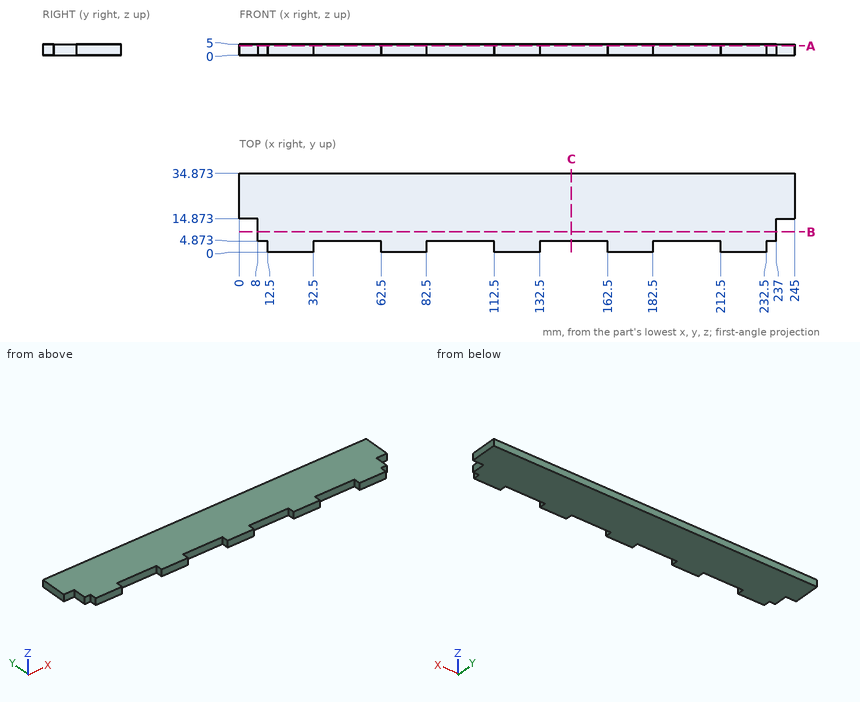
Source: three-view drawing plus pictorial views. Frame: mm from the lowest corner of the part. Give positions to 0.01 mm unless a question says otherwise; leave off trailing zeros. Loops run counter-clockwise (first coordinate to the right, second up) from the corner with the lowest first, then second, coordinate; pieces in that order, holes last.
1) Contact query for flat-ended pins moving along their axis: pin 1 (1.5 mm diameter, centred on y = 2, z = 2.5, fed in from -X); pin 2 (3 mm diameter, centred on x = 147, z = 2, fed in from -Y); pin 3 (2.5 mm diameter, centred on y = 8.5, z = 3, fed in from +X). Output: stop coordinate, or through.
A:
pin 1: stops at x = 12.5
pin 2: stops at y = 4.87
pin 3: stops at x = 237
2) Line query: L1, parallel to Y at x = 40.5, z = 4.15; L2, parallel to X at y = 14, z = 4.35. Output: solid intervals per line, ascending.
A:
L1: y = 4.87 to 34.87
L2: x = 8 to 237
3) Section query A-A on z = 4.2. Return the cut outline in (x, y), and give its area (3 significant figures).
A:
outline: (0, 14.87) - (8, 14.87) - (8, 4.87) - (12.5, 4.87) - (12.5, 0) - (32.5, 0) - (32.5, 4.87) - (62.5, 4.87) - (62.5, 0) - (82.5, 0) - (82.5, 4.87) - (112.5, 4.87) - (112.5, 0) - (132.5, 0) - (132.5, 4.87) - (162.5, 4.87) - (162.5, 0) - (182.5, 0) - (182.5, 4.87) - (212.5, 4.87) - (212.5, 0) - (232.5, 0) - (232.5, 4.87) - (237, 4.87) - (237, 14.87) - (245, 14.87) - (245, 34.87) - (0, 34.87) - close
area: 7,680 mm2
4) Section query C-C on x = 146.5. Return the cut outline in (y, z).
A:
outline: (4.87, 0) - (34.87, 0) - (34.87, 5) - (4.87, 5) - close
5) Section query B-B on y = 9. Return the cut outline in (x, z), and give its area (4 significant figures).
A:
outline: (8, 0) - (237, 0) - (237, 5) - (8, 5) - close
area: 1,145 mm2
